```python
from build123d import *

# Parameters (mm, degrees)
BOSS_EXTRUDE13_START = 6
BOSS_EXTRUDE13_DEPTH = 6
BOSS_EXTRUDE14_DEPTH = 12
SKETCH2_19_R         = 10.418590799
SKETCH2_19_R_2       = 2.65
BOSS_EXTRUDE15_DEPTH = 6
CUT_EXTRUDE1_START   = -6
CUT_EXTRUDE1_DEPTH   = 6
CUT_EXTRUDE2_START   = -12
CUT_EXTRUDE2_DEPTH   = 6
CUT_EXTRUDE4_DEPTH   = 6
SKETCH6_R            = 1.575
CUT_EXTRUDE5_DEPTH   = 227.459741668


# Read off the part's stored shape, not the designer's step: Cut-Extrude2
with BuildPart() as part:
    # Sketch2 → Boss-Extrude13 (new body)
    with BuildSketch(Plane.XY.offset(BOSS_EXTRUDE13_START)):
        with BuildLine():
            ThreePointArc((173.212265813, 14.190949605), (163.177749116, 10.034516697), (159.021316208, 0))
            Line((159.021316208, 0), (170.562265813, 0))
            ThreePointArc((170.562265813, 0), (171.338432843, 1.87383297), (173.212265813, 2.65))
            Line((173.212265813, 2.65), (173.212265813, 14.190949605))
        make_face()
        with BuildLine():
            Line((170.562265813, 0), (159.021316208, 0))
            ThreePointArc((159.021316208, 0), (163.177749116, -10.034516697), (173.212265813, -14.190949605))
            Line((173.212265813, -14.190949605), (173.212265813, -2.65))
            ThreePointArc((173.212265813, -2.65), (171.338432843, -1.87383297), (170.562265813, 0))
        make_face()
        with BuildLine():
            ThreePointArc((187.403215418, 0), (183.634025716, 9.63171694), (174.328689217, 14.146966087))
            ThreePointArc((174.328689217, 14.146966087), (173.77091055, 14.179949462), (173.212265813, 14.190949605))
            Line((173.212265813, 14.190949605), (173.212265813, 2.65))
            ThreePointArc((173.212265813, 2.65), (175.086098783, 1.87383297), (175.862265813, 0))
            Line((175.862265813, 0), (187.403215418, 0))
        make_face()
        with BuildLine():
            ThreePointArc((173.212265813, -14.190949605), (173.77091055, -14.179949462), (174.328689217, -14.146966087))
            ThreePointArc((174.328689217, -14.146966087), (183.634025716, -9.63171694), (187.403215418, 0))
            Line((187.403215418, 0), (175.862265813, 0))
            ThreePointArc((175.862265813, 0), (175.086098783, -1.87383297), (173.212265813, -2.65))
            Line((173.212265813, -2.65), (173.212265813, -14.190949605))
        make_face()
        with BuildLine():
            ThreePointArc((173.212265813, 14.190949605), (163.177749116, 10.034516697), (159.021316208, 0))
            Line((159.021316208, 0), (170.562265813, 0))
            ThreePointArc((170.562265813, 0), (171.338432843, 1.87383297), (173.212265813, 2.65))
            Line((173.212265813, 2.65), (173.212265813, 14.190949605))
        make_face()
        with BuildLine():
            Line((170.562265813, 0), (159.021316208, 0))
            ThreePointArc((159.021316208, 0), (163.177749116, -10.034516697), (173.212265813, -14.190949605))
            Line((173.212265813, -14.190949605), (173.212265813, -2.65))
            ThreePointArc((173.212265813, -2.65), (171.338432843, -1.87383297), (170.562265813, 0))
        make_face()
        with BuildLine():
            ThreePointArc((187.403215418, 0), (183.634025716, 9.63171694), (174.328689217, 14.146966087))
            ThreePointArc((174.328689217, 14.146966087), (173.77091055, 14.179949462), (173.212265813, 14.190949605))
            Line((173.212265813, 14.190949605), (173.212265813, 2.65))
            ThreePointArc((173.212265813, 2.65), (175.086098783, 1.87383297), (175.862265813, 0))
            Line((175.862265813, 0), (187.403215418, 0))
        make_face()
        with BuildLine():
            ThreePointArc((173.212265813, -14.190949605), (173.77091055, -14.179949462), (174.328689217, -14.146966087))
            ThreePointArc((174.328689217, -14.146966087), (183.634025716, -9.63171694), (187.403215418, 0))
            Line((187.403215418, 0), (175.862265813, 0))
            ThreePointArc((175.862265813, 0), (175.086098783, -1.87383297), (173.212265813, -2.65))
            Line((173.212265813, -2.65), (173.212265813, -14.190949605))
        make_face()
    extrude(amount=BOSS_EXTRUDE13_DEPTH)

    # Sketch2<18> → Boss-Extrude14 (add)
    with BuildSketch(Plane.XY):
        with BuildLine():
            add(Edge.make_bspline(
                [(216.328689217, 10.366667201), (213.353925458, 10.66477506), (206.696816501, 11.318389968), (196.26008685, 12.293724806), (185.235415917, 13.263427762), (177.892295007, 13.865740213), (174.328689217, 14.146966087)],
                knots=[0.137765812, 0.137765812, 0.137765812, 0.137765812, 0.152428309, 0.170571841, 0.189174522, 0.206706183, 0.206706183, 0.206706183, 0.206706183], degree=3))
            ThreePointArc((174.328689217, 14.146966087), (183.634025716, 9.63171694), (187.403215418, 0))
            Line((187.403215418, 0), (204.87123106, 0))
            ThreePointArc((204.87123106, 0), (207.922765654, 7.367056204), (215.289821859, 10.418590799))
            ThreePointArc((215.289821859, 10.418590799), (215.809903931, 10.405601803), (216.328689217, 10.366667201))
        make_face()
        with BuildLine():
            ThreePointArc((187.403215418, 0), (183.634025716, -9.63171694), (174.328689217, -14.146966087))
            add(Edge.make_bspline(
                [(174.328689217, -14.146966087), (177.892295007, -13.865740213), (185.235415917, -13.263427762), (196.26008685, -12.293724806), (206.696816501, -11.318389968), (213.353925458, -10.66477506), (216.328689217, -10.366667201)],
                knots=[0.793293817, 0.793293817, 0.793293817, 0.793293817, 0.810825478, 0.829428159, 0.847571691, 0.862234188, 0.862234188, 0.862234188, 0.862234188], degree=3))
            ThreePointArc((216.328689217, -10.366667201), (215.809903931, -10.405601803), (215.289821859, -10.418590799))
            ThreePointArc((215.289821859, -10.418590799), (207.922765654, -7.367056204), (204.87123106, 0))
            Line((204.87123106, 0), (187.403215418, 0))
        make_face()
        with BuildLine():
            add(Edge.make_bspline(
                [(216.328689217, 10.366667201), (213.353925458, 10.66477506), (206.696816501, 11.318389968), (196.26008685, 12.293724806), (185.235415917, 13.263427762), (177.892295007, 13.865740213), (174.328689217, 14.146966087)],
                knots=[0.137765812, 0.137765812, 0.137765812, 0.137765812, 0.152428309, 0.170571841, 0.189174522, 0.206706183, 0.206706183, 0.206706183, 0.206706183], degree=3))
            ThreePointArc((174.328689217, 14.146966087), (183.634025716, 9.63171694), (187.403215418, 0))
            Line((187.403215418, 0), (204.87123106, 0))
            ThreePointArc((204.87123106, 0), (207.922765654, 7.367056204), (215.289821859, 10.418590799))
            ThreePointArc((215.289821859, 10.418590799), (215.809903931, 10.405601803), (216.328689217, 10.366667201))
        make_face()
        with BuildLine():
            ThreePointArc((187.403215418, 0), (183.634025716, -9.63171694), (174.328689217, -14.146966087))
            add(Edge.make_bspline(
                [(174.328689217, -14.146966087), (177.892295007, -13.865740213), (185.235415917, -13.263427762), (196.26008685, -12.293724806), (206.696816501, -11.318389968), (213.353925458, -10.66477506), (216.328689217, -10.366667201)],
                knots=[0.793293817, 0.793293817, 0.793293817, 0.793293817, 0.810825478, 0.829428159, 0.847571691, 0.862234188, 0.862234188, 0.862234188, 0.862234188], degree=3))
            ThreePointArc((216.328689217, -10.366667201), (215.809903931, -10.405601803), (215.289821859, -10.418590799))
            ThreePointArc((215.289821859, -10.418590799), (207.922765654, -7.367056204), (204.87123106, 0))
            Line((204.87123106, 0), (187.403215418, 0))
        make_face()
    extrude(amount=BOSS_EXTRUDE14_DEPTH)

    # Sketch2<19> → Boss-Extrude15 (add)
    with BuildSketch(Plane.XY):
        with Locations((215.289821859, 0)):
            Circle(SKETCH2_19_R)
        with Locations((215.289821859, 0)):
            Circle(SKETCH2_19_R_2, mode=Mode.SUBTRACT)
    extrude(amount=BOSS_EXTRUDE15_DEPTH)

    # Sketch3 → Cut-Extrude1 (cut)
    with BuildSketch(Plane.XY.offset(12).offset(CUT_EXTRUDE1_START)):
        with BuildLine():
            ThreePointArc((174.305087765, -13.847895909), (159.321316208, 0), (174.305087765, 13.847895909))
            Line((174.305087765, 13.847895909), (176.307152097, 13.989700975))
            add(Edge.make_bspline(
                [(176.307152097, 13.989700975), (175.647694257, 14.042496099), (174.988206638, 14.094919544), (174.328689217, 14.146966087)],
                knots=[0.203461594, 0.203461594, 0.203461594, 0.203461594, 0.206706183, 0.206706183, 0.206706183, 0.206706183], degree=3))
            ThreePointArc((174.328689217, 14.146966087), (159.021316208, 0), (174.328689217, -14.146966087))
            add(Edge.make_bspline(
                [(174.328689217, -14.146966087), (174.985934365, -14.095098863), (175.643149915, -14.04285733), (176.300335892, -13.990246656)],
                knots=[0.793293817, 0.793293817, 0.793293817, 0.793293817, 0.796527227, 0.796527227, 0.796527227, 0.796527227], degree=3))
            Line((176.300335892, -13.990246656), (174.305087765, -13.847895909))
        make_face()
        with BuildLine():
            add(Edge.make_bspline(
                [(216.328689217, 10.366667201), (215.491519854, 10.450561851), (214.654303032, 10.533983064), (213.817038746, 10.616925102)],
                knots=[0.137765812, 0.137765812, 0.137765812, 0.137765812, 0.141892188, 0.141892188, 0.141892188, 0.141892188], degree=3))
            ThreePointArc((213.817038746, 10.616925102), (204.57123106, 0), (213.817038746, -10.616925102))
            add(Edge.make_bspline(
                [(213.817038746, -10.616925102), (214.654303032, -10.533983064), (215.491519854, -10.450561851), (216.328689217, -10.366667201)],
                knots=[0.858107812, 0.858107812, 0.858107812, 0.858107812, 0.862234188, 0.862234188, 0.862234188, 0.862234188], degree=3))
            ThreePointArc((216.328689217, -10.366667201), (204.87123106, 0), (216.328689217, 10.366667201))
        make_face()
    extrude(amount=CUT_EXTRUDE1_DEPTH, mode=Mode.SUBTRACT)

    # Cut-Extrude2 outline → Cut-Extrude2 (cut)
    with BuildSketch(Plane.XY.offset(12).offset(CUT_EXTRUDE2_START)):
        with BuildLine():
            ThreePointArc((174.328689217, 14.146966087), (175.06538064, 14.06943553), (175.797022727, 13.953568804))
            Line((175.797022727, 13.953568804), (176.307152091, 13.989700975))
            add(Edge.make_bspline(
                [(176.307152091, 13.989700975), (175.647694253, 14.042496099), (174.988206637, 14.094919544), (174.328689217, 14.146966087)],
                knots=[0.203461594, 0.203461594, 0.203461594, 0.203461594, 0.206706183, 0.206706183, 0.206706183, 0.206706183], degree=3))
        make_face()
        with BuildLine():
            Line((176.300335892, -13.990246656), (175.794024244, -13.95412391))
            ThreePointArc((175.794024244, -13.95412391), (175.063868969, -14.069634552), (174.328689217, -14.146966087))
            add(Edge.make_bspline(
                [(174.328689217, -14.146966087), (174.985934365, -14.095098863), (175.643149916, -14.04285733), (176.300335892, -13.990246656)],
                knots=[0.793293817, 0.793293817, 0.793293817, 0.793293817, 0.796527227, 0.796527227, 0.796527227, 0.796527227], degree=3))
        make_face()
    extrude(amount=CUT_EXTRUDE2_DEPTH, mode=Mode.SUBTRACT)

    # Sketch5 → Cut-Extrude4 (cut)
    with BuildSketch(Plane(origin=(0, 0, 0), x_dir=(-1, 0, 0), z_dir=(0, 0, -1))):
        with BuildLine():
            add(Edge.make_bspline(
                [(-177.264696566, -13.912779214), (-176.943250082, -13.938689614), (-176.621796525, -13.964512296), (-176.300335892, -13.990246656)],
                knots=[0.860652575, 0.860652575, 0.860652575, 0.860652575, 0.862234188, 0.862234188, 0.862234188, 0.862234188], degree=3))
            Line((-176.300335892, -13.990246656), (-175.794024244, -13.95412391))
            ThreePointArc((-175.794024244, -13.95412391), (-187.403215336, -0.001524716), (-175.797022727, 13.953568805))
            Line((-175.797022727, 13.953568805), (-176.307152091, 13.989700975))
            add(Edge.make_bspline(
                [(-176.307152091, 13.989700975), (-176.626340558, 13.964147265), (-176.945522049, 13.93850648), (-177.264696566, 13.912779214)],
                knots=[0.137765812, 0.137765812, 0.137765812, 0.137765812, 0.139336246, 0.139336246, 0.139336246, 0.139336246], degree=3))
            ThreePointArc((-177.264696566, 13.912779214), (-187.703215418, 0), (-177.264696566, -13.912779214))
        make_face()
    extrude(amount=-CUT_EXTRUDE4_DEPTH, mode=Mode.SUBTRACT)

    # Sketch6 → Cut-Extrude5 (cut, through all)
    with BuildSketch(Plane.XY.offset(12)):
        with Locations((192.082086145, 5.4)):
            Circle(SKETCH6_R)
        with Locations((192.082086145, -5.4)):
            Circle(SKETCH6_R)
    extrude(amount=-CUT_EXTRUDE5_DEPTH, mode=Mode.SUBTRACT)


solid = part.part
```
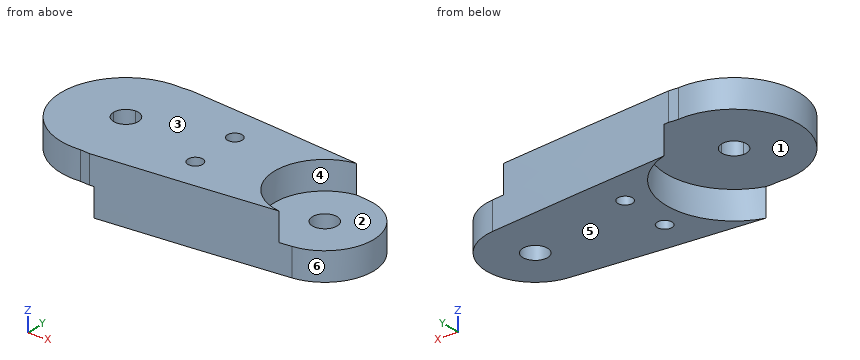
Can you work these out from the model? Positions are in its coordinate system, mm. Face numbers are marked on the shaded views. A direction names the side the tool comes from. Coordinates: 2 decimals unless noted, no trailing zeros. Order: outer loops, then holes, each group sorted by start corner. A loop starts at its lowest first (then second) coordinate and runs counter-clockwise, first axis right, second up.
1. If we section it at C-C (z = 2.5): Give the number of separate pieces and of enclosed holes in the cut face, then the cut area to 3 significant figures.
2. If we section it at D-D (y = 9): Please give me the cut outline in (x, z), then the cut area to 3 significant figures.
3. If we section it at A-A (x = 217): Please give me the cut outline in (y, z), then the cut area to 3 significant figures.
4. I'm going to push flat-ended pins straight in: pin 1 (8.5 mm diameter, centred on x = 173.5, y = -5.5, fed in from -Z); pin 2 (2.5 mm diameter, centred on x = 192.08, y = 5.4, fed in from +Z); pin 3 (3 mm diameter, centred on x = 204, z = 8, fed in from +Y); pin 4 (2 mm diameter, centred on y = -3, z = 9, fed in from +X). Where does each tip first touch, or does it pass through?
5. Thinking about a two-plate mould opening in Y: for the marked faces 4, 5 and 6, which applies, +Y half, -Y half, draft (parallel to the pull), parting line (faces both ways), or undercut?
6. For the marked faces 1, 2 and 3, which set-ups out of +Z, -Z, +X, -X, +Y, -Y let a thin tool reach every point of the face, with its end or its side?
7. If we section it at B-B (y = 5.4): Please give me the cut outline in (x, z), then the cut area to 3 significant figures.
8. I need wall thicknesses on line 1 (Z direction, x = 163, y = -4); line 2 (Z direction, x = 214, y = -3.5); line 3 (Y direction, x = 209.5, z = 11). Which ranges of each line are inside material? Lowest first, please.
Entries:
1. separate pieces: 1
1. enclosed holes: 3
1. area: 851 mm2
2. outline: (162.63, 6) - (184.57, 6) - (184.57, 0) - (220.54, 0) - (220.54, 6) - (209.47, 6) - (209.47, 12) - (162.63, 12) - close
2. area: 497 mm2
3. outline: (-10.28, 0) - (-2.02, 0) - (-2.02, 6) - (-10.28, 6) - close; (2.02, 0) - (10.28, 0) - (10.28, 6) - (2.02, 6) - close
3. area: 99.0 mm2
4. pin 1: stops at z = 6
4. pin 2: passes through
4. pin 3: stops at y = 11.71
4. pin 4: stops at x = 205.35
5. face 4: undercut
5. face 5: draft
5. face 6: parting line
6. face 1: -Z, -X
6. face 2: +Z, +X
6. face 3: +Z, +X, -X, +Y, -Y
7. outline: (160.41, 6) - (186.66, 6) - (186.66, 0) - (190.51, 0) - (190.51, 12) - (160.41, 12) - close; (193.66, 0) - (224.2, 0) - (224.2, 6) - (206.03, 6) - (206.03, 12) - (193.66, 12) - close
7. area: 461 mm2
8. line 1: z = 6 to 12
8. line 2: z = 0 to 6
8. line 3: y = -11.04 to -9.02, 9.02 to 11.04
